```python
from build123d import *

# Parameters (mm, degrees)
EXTRUDE_1_DEPTH     = 1.25
SKETCH_1_3_R        = 2
CUT_EXTRUDE_1_DEPTH = 37.497164572
FILLET_1_R          = 3
EXTRUDE_START       = -1.25
SKETCH_2_R          = 2
EXTRUDE_2_DEPTH     = 1.25
SKETCH_2_5_R        = 1.8
EXTRUDE_5_DEPTH     = 2.5
SKETCH_2_7_R        = 1.8
EXTRUDE_7_DEPTH     = 5
EXTRUDE_8_DEPTH     = 1
EXTRUDE_START_2     = 1
SKETCH_3_3_R        = 2.5
EXTRUDE_9_DEPTH     = 1


with BuildPart() as part:
    # 草图1 → 凸台-拉伸1 (new body)
    with BuildSketch(Plane(origin=(0, 0, 0), x_dir=(0, 0, -1), z_dir=(1, 0, 0))):
        with BuildLine():
            Line((-28.172077255, -4.520836084), (-28.172077255, 1.479163916))
            Line((-28.172077255, 1.479163916), (-24.707975639, 1.479163916))
            ThreePointArc((-24.707975639, 1.479163916), (-31.63617887, 1.479163916), (-28.172077255, -4.520836084))
        make_face()
        with BuildLine():
            Line((-24.707975639, 1.479163916), (-28.172077255, 1.479163916))
            Line((-28.172077255, 1.479163916), (-28.172077255, -4.520836084))
            ThreePointArc((-28.172077255, -4.520836084), (-25.34365013, -3.349263209), (-24.172077255, -0.520836084))
            ThreePointArc((-24.172077255, -0.520836084), (-24.308373949, 0.514440097), (-24.707975639, 1.479163916))
        make_face()
        with BuildLine():
            Line((-3.172077255, 1.479163916), (-24.707975639, 1.479163916))
            ThreePointArc((-24.707975639, 1.479163916), (-24.308373949, 0.514440097), (-24.172077255, -0.520836084))
            ThreePointArc((-24.172077255, -0.520836084), (-25.34365013, -3.349263209), (-28.172077255, -4.520836084))
            Line((-28.172077255, -4.520836084), (-5.969923204, -4.520836084))
            Line((-5.969923204, -4.520836084), (-3.172077255, 1.479163916))
        make_face()
        with BuildLine():
            Line((3.172077255, -1.479163916), (-3.172077255, 1.479163916))
            Line((-3.172077255, 1.479163916), (-3.172077255, -1.479163916))
            ThreePointArc((-3.172077255, -1.479163916), (0, -3.5), (3.172077255, -1.479163916))
        make_face()
        with BuildLine():
            ThreePointArc((3.5, 0), (0.757538649, 3.417036025), (-3.172077255, 1.479163916))
            Line((-3.172077255, 1.479163916), (3.172077255, -1.479163916))
            ThreePointArc((3.172077255, -1.479163916), (3.417036025, -0.757538649), (3.5, 0))
        make_face()
        with BuildLine():
            ThreePointArc((-3.172077255, -1.479163916), (-3.5, 0), (-3.172077255, 1.479163916))
            Line((-3.172077255, 1.479163916), (-5.969923204, -4.520836084))
            Line((-5.969923204, -4.520836084), (-3.172077255, -4.520836084))
            Line((-3.172077255, -4.520836084), (-3.172077255, -1.479163916))
        make_face()
        with BuildLine():
            Line((-3.172077255, -1.479163916), (-3.172077255, 1.479163916))
            ThreePointArc((-3.172077255, 1.479163916), (-3.5, 0), (-3.172077255, -1.479163916))
        make_face()
        with BuildLine():
            Line((-3.172077255, -4.520836084), (-5.969923204, -4.520836084))
            Line((-5.969923204, -4.520836084), (-7.893387964, -8.645719574))
            ThreePointArc((-7.893387964, -8.645719574), (-4.014873487, -8.609923977), (-1.549233455, -11.604047406))
            Line((-1.549233455, -11.604047406), (3.172077255, -1.479163916))
            ThreePointArc((3.172077255, -1.479163916), (0, -3.5), (-3.172077255, -1.479163916))
            Line((-3.172077255, -1.479163916), (-3.172077255, -4.520836084))
        make_face()
        with BuildLine():
            ThreePointArc((-1.549233455, -11.604047406), (-4.014873487, -8.609923977), (-7.893387964, -8.645719574))
            Line((-7.893387964, -8.645719574), (-9.088732919, -11.209145102))
            Line((-9.088732919, -11.209145102), (-2.74457841, -14.167472935))
            Line((-2.74457841, -14.167472935), (-1.549233455, -11.604047406))
        make_face()
        with BuildLine():
            Line((-9.088732919, -11.209145102), (-7.893387964, -8.645719574))
            ThreePointArc((-7.893387964, -8.645719574), (-8.299375187, -16.50572276), (-1.416655664, -12.688309019))
            ThreePointArc((-1.416655664, -12.688309019), (-1.449923081, -12.14214052), (-1.549233455, -11.604047406))
            Line((-1.549233455, -11.604047406), (-2.74457841, -14.167472935))
            Line((-2.74457841, -14.167472935), (-9.088732919, -11.209145102))
        make_face()
    extrude(amount=EXTRUDE_1_DEPTH)

    # 草图1<3> → 切除-拉伸1 (cut, through all)
    with BuildSketch(Plane(origin=(0, 0, 0), x_dir=(0, 0, -1), z_dir=(1, 0, 0))):
        with Locations((-28.172077255, -0.520836084)):
            Circle(SKETCH_1_3_R)
        Circle(SKETCH_1_3_R)
        with Locations((-5.916655664, -12.688309019)):
            Circle(SKETCH_1_3_R)
    extrude(amount=CUT_EXTRUDE_1_DEPTH, mode=Mode.SUBTRACT)

    # 圆角1
    # the kernel refuses this fillet: 3 mm, written as the material it adds along each edge
    with BuildSketch(Plane(origin=(0, -11.604047406, 1.549233455), x_dir=(0, 0.9063077870366663, -0.4226182617406644), z_dir=(1, 0, 0))) as fillet_1_piece_1:
        with BuildLine():
            CenterArc((0.913230262, -3), FILLET_1_R, 90, 29.926434867)
            Line((-0.583432693, -0.4), (-0.613365952, -0.348))
            ThreePointArc((-0.613365952, -0.348), (-0.317772106, -0.161995545), (-0.037712362, 0.046666667))
            Line((-0.037712362, 0.046666667), (0, 0.06))
            Line((0, 0.06), (0.913230262, 0.06))
            Line((0.913230262, 0.06), (0.913230262, 0))
        make_face()
    extrude(amount=1.25)
    with BuildSketch(Plane(origin=(0, 1.479163916, 3.172077255), x_dir=(0, 0, 1), z_dir=(1, 0, 0))) as fillet_1_piece_2:
        with BuildLine():
            CenterArc((1.538240209, -3), FILLET_1_R, 90, 46.440922497)
            Line((-0.635752466, -0.932693577), (-0.67923232, -0.891347449))
            ThreePointArc((-0.67923232, -0.891347449), (-0.329607023, -0.458350724), (-0.054378467, 0.025357096))
            Line((-0.054378467, 0.025357096), (0, 0.06))
            Line((0, 0.06), (1.538240209, 0.06))
            Line((1.538240209, 0.06), (1.538240209, 0))
        make_face()
    extrude(amount=1.25)
    with BuildSketch(Plane(origin=(0, 1.479163916, 24.707975639), x_dir=(0, 0.7902368852402469, 0.6128014892326821), z_dir=(1, 0, 0))) as fillet_1_piece_3:
        with BuildLine():
            CenterArc((1.49141536, -2.972297887), FILLET_1_R, 97.792345701, 44.415308597)
            Line((-0.879295296, -1.133893419), (-0.926709509, -1.09712533))
            Line((-0.926709509, -1.09712533), (-0.047414213, 0.036768089))
            Line((-0.047414213, 0.036768089), (0.008134993, 0.059445958))
            ThreePointArc((0.008134993, 0.059445958), (0.542332858, 0.023063849), (1.076530723, 0.059445958))
            Line((1.076530723, 0.059445958), (1.084665716, 0))
        make_face()
    extrude(amount=1.25)
    with BuildSketch(Plane(origin=(0, -4.520836084, 5.969923204), x_dir=(0, 0, 1), z_dir=(1, 0, 0))) as fillet_1_piece_4:
        with BuildLine():
            CenterArc((4.704586321, 3), FILLET_1_R, 157.978087479, 112.021912521)
            Line((1.923464761, 4.12488349), (1.867842329, 4.14738116))
            ThreePointArc((1.867842329, 4.14738116), (0.907353913, 2.087798841), (-0.054378467, 0.025357096))
            Line((-0.054378467, 0.025357096), (0, -0.06))
            Line((0, -0.06), (4.704586321, -0.06))
            Line((4.704586321, -0.06), (4.704586321, 0))
        make_face()
    extrude(amount=1.25)

    # 草图2 → 凸台-拉伸2 (add)
    with BuildSketch(Plane(origin=(1.25, 0, 0), x_dir=(0, 0, -1), z_dir=(1, 0, 0)).offset(EXTRUDE_START)):
        Circle(SKETCH_2_R)
        with Locations((-5.916655664, -12.688309019)):
            Circle(SKETCH_2_R)
        with Locations((-28.172077255, -0.520836084)):
            Circle(SKETCH_2_R)
    extrude(amount=EXTRUDE_2_DEPTH)

    # 草图2<5> → 凸台-拉伸5 (add)
    with BuildSketch(Plane(origin=(1.25, 0, 0), x_dir=(0, 0, -1), z_dir=(1, 0, 0))):
        with Locations((-28.172077255, -0.520836084)):
            Circle(SKETCH_2_5_R)
        Circle(SKETCH_2_5_R)
    extrude(amount=EXTRUDE_5_DEPTH)

    # 草图2<7> → 凸台-拉伸7 (add)
    with BuildSketch(Plane(origin=(1.25, 0, 0), x_dir=(0, 0, -1), z_dir=(1, 0, 0))):
        with Locations((-5.916655664, -12.688309019)):
            Circle(SKETCH_2_7_R)
    extrude(amount=EXTRUDE_7_DEPTH)

    # 草图3 → 凸台-拉伸8 (add)
    with BuildSketch(Plane(origin=(1.25, 0, 0), x_dir=(0, 0, -1), z_dir=(1, 0, 0))):
        with BuildLine():
            ThreePointArc((-12.5, -1.520836084), (-12.939339828, -0.460175912), (-14, -0.020836084))
            Line((-14, -0.020836084), (-14, -3.020836084))
            ThreePointArc((-14, -3.020836084), (-12.939339828, -2.581496256), (-12.5, -1.520836084))
        make_face()
        with BuildLine():
            Line((-14, -3.020836084), (-14, -0.020836084))
            ThreePointArc((-14, -0.020836084), (-15.5, -1.520836084), (-14, -3.020836084))
        make_face()
    extrude(amount=EXTRUDE_8_DEPTH)

    # 草图3<3> → 凸台-拉伸9 (add)
    with BuildSketch(Plane(origin=(1.25, 0, 0), x_dir=(0, 0, -1), z_dir=(1, 0, 0)).offset(EXTRUDE_START_2)):
        with Locations((-14, -1.520836084)):
            Circle(SKETCH_3_3_R)
    extrude(amount=EXTRUDE_9_DEPTH)

    # 镜向1: part across plane


with BuildPart() as part_1:
    add(part.part)
    add(part.part.mirror(Plane.ZY))


solid = part_1.part
```
CAD build for the part. Positions are in the model's coordinates, mm. A direction names the side the tool comes from. Coordinates: 2 decimals unless noted, no trailing zeros. Order: outer loops, then holes, each group sorted by start corner. A loop starts at its lowest first (then second) coordinate and runs counter-clockwise, first axis right, second up. Notation, with made-up numbers: (-8.75, 76.5) -> (9.25, 76.5) arc R25 cw to (9.25, 94.5) -> close; hole circle Ø9 at (30, 55). An arc over 180 degrees is marked (long way). Use one line per item in the form item = value. Start each with the question number.
1) Drop flat-ended pins along their axis: pin 1 (1.8 mm diameter, centred on y = 0, z = -0.5, fed in from -X); pin 2 (2 mm diameter, centred on x = -3, z = 4, fed in from +Y); pin 3 (1 mm diameter, centred on x = 0.5, z = 19, fed in from -Y); pin 4 (4 mm diameter, centred on x = -5, y = -6, fed in from -Z). Give the stop position or say it passes through.
2) Band-saw the part on C-C on z = 0. Give the cut face in (x, y), then the cut area to 3 significant figures.
3) Band-saw the part on B-B on x = 0.5. Give the cut face in (y, z).
4) Drill centre lines: L1, parallel to X at y = -11.5, z = 10; L2, parallel to X at y = -1.5, z = 28.5; L3, parallel to Y at x = -0.5, z = 6.5. Where is each one in solid material? Low to high. Write a range as [from, to].
5) Tool access for faces 4 (the cylindrical face through (2.743, -1.411, 16.498)), 5 (the flat face through (2.25, -3, 13)), 6 (the cylindrical face through (-2.743, -1.411, 16.498)): list every direction of +Z, -Z, +X, -X, +Y, -Y with a clear straight run to the whole face (end or side of a thin tool).
6) Band-saw the part on D-D on y = -9.5. Give the cut face in (x, z), then the cut area to 3 significant figures.
7) Pull direction Z, two halves, no side cores. Call faces 1 (the cylindrical face through (3.715, -14.285, 5.086)), 2 (the cylindrical face through (-2.482, 0.541, -1.717)), 3 (the flat face through (3.75, 0, 0)): +Z half, -Z half, draft (parallel to the pull), parting line (faces both ways), or undercut.
8) Band-saw the part on A-A on z = 16. Give the cut face in (x, y), then the cut area to 3 significant figures.
Entries:
q1.pin_1 = -3.75
q1.pin_2 = -11.14
q1.pin_3 = -4.52
q1.pin_4 = through
q2.outline = (-3.75, -1.8) -> (-1.25, -1.8) -> (-1.25, -8.28) -> (1.25, -8.28) -> (1.25, -1.8) -> (3.75, -1.8) -> (3.75, 1.8) -> (1.25, 1.8) -> (1.25, 3.5) -> (-1.25, 3.5) -> (-1.25, 1.8) -> (-3.75, 1.8) -> close
q2.area = 47.5 mm2
q3.outline = (-12.3, 1.43) arc R3 cw to (-10.78, 1.16) -> (-1.48, -3.17) arc R3.5 ccw to (2.41, 2.54) arc R3 cw to (1.48, 4.71) -> (1.48, 23.27) arc R3 cw to (2.34, 25.37) arc R4 ccw (long way) to (-4.52, 28.17) -> (-4.52, 10.67) arc R3 cw to (-8.65, 7.89) arc R4.5 ccw (long way) to start
q4.L1 = [-1.25, 1.25]
q4.L2 = [-3.75, 3.75]
q4.L3 = [-17.15, 1.48]
q5.face_4 = +X
q5.face_5 = none
q5.face_6 = -X
q6.outline = (-1.25, 0.57) -> (1.25, 0.57) -> (1.25, 9.09) -> (-1.25, 9.09) -> close
q6.area = 21.3 mm2
q7.face_1 = parting line
q7.face_2 = undercut
q7.face_3 = draft
q8.outline = (-3.25, -3.02) -> (-2.25, -3.02) -> (-2.25, -0.02) -> (-3.25, -0.02) -> close; (-1.25, -4.52) -> (1.25, -4.52) -> (1.25, 1.48) -> (-1.25, 1.48) -> close; (2.25, -3.02) -> (3.25, -3.02) -> (3.25, -0.02) -> (2.25, -0.02) -> close
q8.area = 21.0 mm2
